from build123d import *

# Parameters (mm, degrees)
SKETCH1_R           = 2.5
BOSS_EXTRUDE1_DEPTH = 1.25


with BuildPart() as part:
    # Sketch1 → Boss-Extrude1 (new, symmetric)
    with BuildSketch(Plane.XY):
        Polygon((0, 0), (65, 0), (65, 16), (16, 16), (16, 65), (0, 65), align=None)
        with Locations((25, 8)):
            Circle(SKETCH1_R, mode=Mode.SUBTRACT)
        with Locations((50, 8)):
            Circle(SKETCH1_R, mode=Mode.SUBTRACT)
        with Locations(Location((8, 50, 0), (0, 0, 180))):
            Circle(SKETCH1_R, mode=Mode.SUBTRACT)
        with Locations(Location((8, 25, 0), (0, 0, 180))):
            Circle(SKETCH1_R, mode=Mode.SUBTRACT)
    extrude(amount=BOSS_EXTRUDE1_DEPTH, both=True)


solid = part.part
The listing builds one solid part. Answer for the finished solid, in the listing's coordinates (mm). A direction names the side the tool comes from. Coordinates: 2 decimals unless noted, no trailing zeros. Loops run counter-clockwise (first coordinate to the right, second up) from the corner with the lowest first, then second, coordinate; pieces in that order, holes last. Notation, with made-up numbers: (-14, 34.5) -> (-4, 34.5) arc R8 ccw to (-4, 48.5) -> close; hole circle Ø9 at (50.25, 58). An arc over 180 degrees is marked (long way). Answer in a Markdown table with one row per item. Add a question column.
1. The part is cut by section A-A, the plane x = 8. Write down the section's boundary in (y, z).
2. The part is cut by section B-B, the plane y = 9.5. Write down the section's boundary in (x, z), then the cut area to 4 significant figures.
3. A flat-ended cylindrical pin translates along its axis: P1, Ø8, axis at x = 51, y = 21, coming from the -Z side. Find the tip coordinate at first contact, or state that the pin passes through.
4. Determine the mould class of faces 3 (the cylindrical face through (8.54, 52.44, -0.02)), 4 (the flat face through (25, 11, 1.25)), 5 (the flat face through (16, 40, 0)) for opening direction X: +X half, -X half, draft (parallel to the pull), parting line (faces both ways), or undercut.
5. The part is cut by section C-C, the plane y = 50. Write down the section's boundary in (x, z).
6. Consider line 1 (Y direction, x = 8, z = -0.6); line 2 (Y direction, x = 50, z = 0.6). Determine where each line is inside the solid, lowest interval first. Write a range as [from, to].
7. For faces 1 (the cylindrical face through (24.46, 5.56, -0.02)), 2 (the flat face through (41, 16, 0)), determine the directions among +Z, -Z, +X, -X, +Y, -Y from which every point of the face is accessible in a straight line to the end or side of a thin tool.
Answer below:
| question | item | result |
|---|---|---|
| 1 | outline | (0, -1.25) -> (22.5, -1.25) -> (22.5, 1.25) -> (0, 1.25) -> close; (27.5, -1.25) -> (47.5, -1.25) -> (47.5, 1.25) -> (27.5, 1.25) -> close; (52.5, -1.25) -> (65, -1.25) -> (65, 1.25) -> (52.5, 1.25) -> close |
| 2 | outline | (0, -1.25) -> (23, -1.25) -> (23, 1.25) -> (0, 1.25) -> close; (27, -1.25) -> (48, -1.25) -> (48, 1.25) -> (27, 1.25) -> close; (52, -1.25) -> (65, -1.25) -> (65, 1.25) -> (52, 1.25) -> close |
| 2 | area | 142.5 mm2 |
| 3 | P1 | through |
| 4 | face 3 | undercut |
| 4 | face 4 | draft |
| 4 | face 5 | +X half |
| 5 | outline | (0, -1.25) -> (5.5, -1.25) -> (5.5, 1.25) -> (0, 1.25) -> close; (10.5, -1.25) -> (16, -1.25) -> (16, 1.25) -> (10.5, 1.25) -> close |
| 6 | line 1 | [0, 22.5], [27.5, 47.5], [52.5, 65] |
| 6 | line 2 | [0, 5.5], [10.5, 16] |
| 7 | face 1 | +Z, -Z |
| 7 | face 2 | +Z, -Z, +X, +Y |
